For this review, take the finished solid that the model builds, in its own axes (mm). Face numbers are marked on the shaded views. A direction names the side the tool comes from. Give positions to 0.01 mm unless a question says otherwise; leave off trailing zeros. Write each loop counter-clockwise with the first axis right and the second up, starting at its lowest first coordinate (ties: lowest second). Pieces come first, ordered by that corner, then holes. Notation, with made-up numbers: M 42.25,-37.5 L 47.25,-37.5 A6 ccw 47.25,-27.5 Z; hole C 63,38 d10. An arc over 180 degrees is marked long. One line per item, written item: value. Start each with the question number.
Item 1: Consider section A-A, the plane x = 0. Write out the cut boundary in (y, z).
Item 2: Consider section B-B, the plane z = -3.5. Write out the cut boundary in (x, y).
Item 3: Tool access review of the marked faces 1, 2, 3, 4 and 5: name each direction out of +Z, -Z, +X, -X, +Y, -Y from which nothing blocks a thin tool from reaching the whole face with its end or side.
Item 4: Clearance check with flat-ended pins moving along their axes: pin 1 Ø5 at (x, z) = (-16.5, 3.5) entering from +Y; pin 2 Ø2 at (x, y) = (10.5, 8.5) entering from +Z; pin 3 Ø12 at (y, z) = (-5.5, -33.5) entering from -X; pin 4 Ø5 at (y, z) = (16, 6) entering from +X. State where each tip first meets the part, or that it passes through.
Item 5: To check wall thickness, follow probe 1 along Z at (x, y) = (8.5, -0.5); probe 2 along X at (y, z) = (8.5, 1); probe 3 along Y at (x, z) = (3, -40.5). State the ranges of each line that lie inside material, in increasing order.
Item 6: Consider section C-C, the plane y = 21.5. Write out the cut boundary in (x, z).
Item 7: Consider section D-D, the plane x = 15. Write out the cut boundary in (y, z).
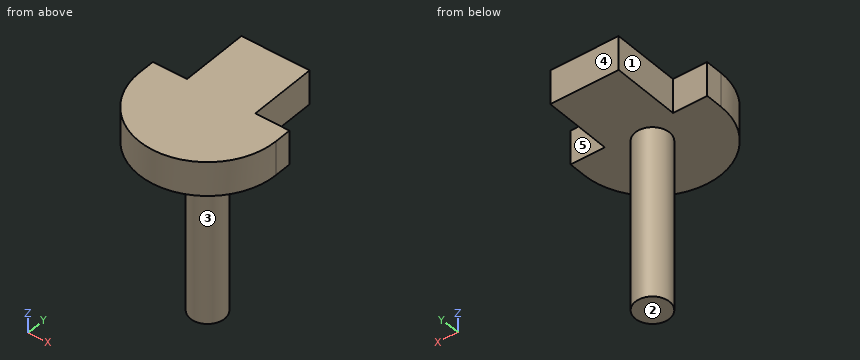
```python
from build123d import *

# Parameters (mm, degrees)
BOSS_EXTRU_1_DEPTH = 10
ESQUISSE2_R        = 5
BOSS_EXTRU_2_DEPTH = 50


with BuildPart() as part:
    # Esquisse1 → Boss.-Extru.1 (new body)
    with BuildSketch(Plane.XY):
        with BuildLine():
            Line((-20, 0), (-20, 5))
            Line((-20, 5), (-10, 5))
            Line((-10, 5), (-10, 25))
            Line((-10, 25), (10, 25))
            Line((10, 25), (10, 5))
            Line((10, 5), (20, 5))
            Line((20, 5), (20, 0))
            ThreePointArc((20, 0), (0, -20), (-20, 0))
        make_face()
    extrude(amount=BOSS_EXTRU_1_DEPTH)

    # Esquisse2 → Boss.-Extru.2 (add)
    with BuildSketch(Plane(origin=(0, 0, 0), x_dir=(-1, 0, 0), z_dir=(0, 0, -1))):
        Circle(ESQUISSE2_R)
    extrude(amount=BOSS_EXTRU_2_DEPTH)


solid = part.part
```
Model answer:
1. outline: M -20,0 L -5,0 L -5,-50 L 5,-50 L 5,0 L 25,0 L 25,10 L -20,10 Z
2. outline: C 0,0 d10
3. face 1: +Z, -Z, -X, +Y
3. face 2: -Z, +X, -X, +Y, -Y
3. face 3: -Z
3. face 4: +Z, -Z, +X, -X, +Y
3. face 5: +Z, -Z, +X, +Y
4. pin 1: stops at y = 5
4. pin 2: stops at z = 10
4. pin 3: stops at x = -5
4. pin 4: stops at x = 10
5. probe 1: z = 0 to 10
5. probe 2: x = -10 to 10
5. probe 3: y = -4 to 4
6. outline: M -10,0 L 10,0 L 10,10 L -10,10 Z
7. outline: M -13.23,0 L 5,0 L 5,10 L -13.23,10 Z
